```python
from build123d import *

# Parameters (mm, degrees)
BOSS_EXTRUDE1_DEPTH = 27.731531852
BOSS_EXTRUDE2_DEPTH = 2.351851852
SKETCH4_R           = 9.144
BOSS_EXTRUDE3_DEPTH = 25.4


with BuildPart() as part:
    # Sketch1 → Boss-Extrude1 (new body)
    with BuildSketch(Plane.XY):
        Polygon((-33.76168, 0), (33.76168, 0), (33.76168, 44.363451852), (6.3246, 44.363451852), (6.3246, 40.426451852), (31.70428, 40.426451852), (31.70428, 2.351851852), (-31.70428, 2.351851852), (-31.70428, 40.426451852), (-6.3246, 40.426451852), (-6.3246, 44.363451852), (-33.76168, 44.363451852), align=None)
    extrude(amount=BOSS_EXTRUDE1_DEPTH)

    # Sketch2 → Boss-Extrude2 (add)
    with BuildSketch(Plane.XY):
        with BuildLine():
            Line((-9.144, 0), (9.144, 0))
            Line((9.144, 0), (9.144, -19.05))
            ThreePointArc((9.144, -19.05), (0, -28.194), (-9.144, -19.05))
            Line((-9.144, -19.05), (-9.144, 0))
        make_face()
    extrude(amount=BOSS_EXTRUDE2_DEPTH)

    # Sketch4 → Boss-Extrude3 (add)
    with BuildSketch(Plane.XY.offset(2.351851852)):
        with Locations((0, -19.05)):
            Circle(SKETCH4_R)
    extrude(amount=BOSS_EXTRUDE3_DEPTH)


solid = part.part
```
Input: part model. Units: mm. Frame: model coordinates. A direction names the side the tool comes from. Coordinates: 2 decimals unless noted, no trailing zeros. Loops run counter-clockwise (first coordinate to the right, second up) from the corner with the lowest first, then second, coordinate; pieces in that order, holes last. Notation, with made-up numbers: (78, 75.5) - (97, 75.5) arc R28 ccw to (97, 96.5) - close; hole circle Ø1 at (55.25, -22.5). An arc over 180 degrees is marked (long way). Answer in a Markdown table with one row per item.
(1) Cut plane A-A on x = -19. Output: boundary loops of the cut face in (y, z), plus the area to 3 significant figures.
Model answer:
| item | result |
|---|---|
| outline | (0, 0) - (2.35, 0) - (2.35, 27.73) - (0, 27.73) - close; (40.43, 0) - (44.36, 0) - (44.36, 27.73) - (40.43, 27.73) - close |
| area | 174 mm² |
(2) Mould query, pull axis X, two halves, no side actions, for faces 6 (the face through (9.144, -9, 1)), 7 (the face through (4.22, -27.16, 13.68)), 8 (the face through (0, 2.352, 14)), 9 (the face through (0, 0, 0)). Classes: pulls with the +X half, pulls with the -X half, needs draft (parallel to the pull), parting line crosses it, or undercut.
Model answer:
| item | result |
|---|---|
| face 6 | pulls with the +X half |
| face 7 | parting line crosses it |
| face 8 | undercut |
| face 9 | needs draft |
(3) Set-up query: faces 1 (the face through (6.325, 42, 14)), 2 (the face through (-33.762, 22, 14)), 3 (the face through (-9.144, -10, 1)), 4 (the face through (-19, 40.426, 14)), 5 (the face through (-20, 44.363, 14)). Return all of +Z, -Z, +X, -X, +Y, -Y with unobstructed straight access to the full face (end or side cutting, diameter ignored); none if empty.
Model answer:
| item | result |
|---|---|
| face 1 | +Z, -Z, +Y |
| face 2 | +Z, -Z, -X, +Y, -Y |
| face 3 | +Z, -Z, -X, -Y |
| face 4 | +Z, -Z |
| face 5 | +Z, -Z, +X, -X, +Y |
(4) Cut plane B-B on y = 36.5. Output: boundary loops of the cut face in (x, z), plus the area to 3 significant figures.
Model answer:
| item | result |
|---|---|
| outline | (-33.76, 0) - (-31.7, 0) - (-31.7, 27.73) - (-33.76, 27.73) - close; (31.7, 0) - (33.76, 0) - (33.76, 27.73) - (31.7, 27.73) - close |
| area | 114 mm² |
(5) Pin query (flat end, axial travel): P1, Ø9, axis at x = 1, y = -5, coming from the +Z side; P2, Ø5, axis at x = 5, z = 9, coming from the +Y side; P3, Ø2.5, axis at y = -10.5, z = 1.5, coming from the -X side; P4, Ø12, axis at x = -18.5, z = 20.5, coming from the -Y side. Return the tip coordinate at first contact, or that it passes through.
Model answer:
| item | result |
|---|---|
| P1 | stops at z = 2.35 |
| P2 | stops at y = 44.36 |
| P3 | stops at x = -9.14 |
| P4 | stops at y = 0 |
(6) Material intervals for L1, parallel to X at y = 25.5, z = 14; L2, parallel to Y at x = -17, z = 3; L3, parallel to X at y = 40.5, z = 19.5, sorted ascending. Write a range as from..to.
Model answer:
| item | result |
|---|---|
| L1 | x = -33.76..-31.7, 31.7..33.76 |
| L2 | y = 0..2.35, 40.43..44.36 |
| L3 | x = -33.76..-6.32, 6.32..33.76 |
(7) Cut plane C-C on z = 21.75. Output: boundary loops of the cut face in (x, y), plus the area to 3 significant figures.
Model answer:
| item | result |
|---|---|
| outline | (-33.76, 0) - (33.76, 0) - (33.76, 44.36) - (6.32, 44.36) - (6.32, 40.43) - (31.7, 40.43) - (31.7, 2.35) - (-31.7, 2.35) - (-31.7, 40.43) - (-6.32, 40.43) - (-6.32, 44.36) - (-33.76, 44.36) - close; circle Ø18.29 at (0, -19.05) |
| area | 794 mm² |
(8) Cut plane D-D on x = 0. Output: boundary loops of the cut face in (y, z), plus the area to 3 significant figures.
Model answer:
| item | result |
|---|---|
| outline | (-28.19, 0) - (2.35, 0) - (2.35, 27.73) - (0, 27.73) - (0, 2.35) - (-9.91, 2.35) - (-9.91, 27.75) - (-28.19, 27.75) - close |
| area | 596 mm² |
